Check sheet for the modelled part. Datum: model origin and axes. Units: mm. A direction names the side the tool comes from. Give positions to 0.01 mm unless a question says otherwise; leave off trailing zeros. Order: outer loops, then holes, each group sorted by start corner. A loop starts at its lowest first (then second) coordinate and runs counter-clockwise, first axis right, second up.
Item 1: Sectioned sample at B-B on y = 45.5. Record the boundary of the cut face in (x, z).
Item 2: Access from +Z, -Z, +X, -X, +Y, -Y to the whole of each face (thin tool, end or side, straight path). Record for faces 1 (the flat face through (-117, 30, 88)), 2 (the flat face through (-110, 2, 59)), 3 (the flat face through (107, 70, -92)), 4 (the flat face through (-107, 70, 92)).
Item 3: Sectioned sample at C-C on x = -12.5. Record the boundary of the cut face in (y, z), and give its area (3 significant figures).
Item 4: Sectioned sample at D-D on z = -6. Record the boundary of the cut face in (x, y).
Item 5: Gauge pin test, flat ends, axial feed: P1, Ø10, axis at x = -89.5, z = -13.5, coming from the +Y side; P2, Ø3, axis at x = 94, z = -15, coming from the -Y side. Record the tip position at first contact, or that the pin passes through.
Item 6: Material ranges on line 1 along X through (y, z) = (3.4, 87.5); line 2 along X through (y, z) = (2, 87); line 3 along Y through (x, z) = (98, 87.5), recorded low to high.
Item 7: Sectioned sample at A-A on z = 61.5. Record the boundary of the cut face in (x, y), and give its area (3 significant figures).
Item 8: Release check for a two-part mould opening along X. For faces 5 (the flat face through (125, 76, 0)), 6 (the flat face through (107, 71, 92)), 7 (the flat face through (115, 0, -73)) record: released by +X, released by -X, zero draft, split by the parting line, or undercut.
from build123d import *

# Parameters (mm, degrees)
BOSS_EXTRUDE1_DEPTH   = 100
BOSS_EXTRUDE1_2_DEPTH = 100
BOSS_EXTRUDE1_3_DEPTH = 100
BOSS_EXTRUDE1_4_DEPTH = 100
SKETCH3_W             = 190
SKETCH3_H             = 5
BOSS_EXTRUDE3_DEPTH   = 250
SKETCH5_R             = 2.5
BOSS_EXTRUDE6_DEPTH   = 5
BOSS_EXTRUDE7_DEPTH   = 45
CUT_EXTRUDE2_REACH    = 197.096
CUT_EXTRUDE3_REACH    = 215.454
CUT_EXTRUDE4_REACH    = 197.096
CUT_EXTRUDE5_REACH    = 215.454


with BuildPart() as part:
    # Sketch1 → Boss-Extrude1 (new body)
    with BuildSketch(Plane(origin=(0, 0, 0), x_dir=(1, 0, 0), z_dir=(0, 1, 0))):
        Polygon((-125, 95), (-125, 80), (-110, 95), align=None)
    extrude(amount=BOSS_EXTRUDE1_DEPTH)



with BuildPart() as body_2:
    # Sketch1 → Boss-Extrude1 2 (new body)
    with BuildSketch(Plane(origin=(0, 0, 0), x_dir=(1, 0, 0), z_dir=(0, 1, 0))):
        Polygon((125, 95), (110, 95), (125, 80), align=None)
    extrude(amount=BOSS_EXTRUDE1_2_DEPTH)


with BuildPart() as body_3:
    # Sketch1 → Boss-Extrude1 3 (new body)
    with BuildSketch(Plane(origin=(0, 0, 0), x_dir=(1, 0, 0), z_dir=(0, 1, 0))):
        Polygon((125, -95), (125, -80), (110, -95), align=None)
    extrude(amount=BOSS_EXTRUDE1_3_DEPTH)


with BuildPart() as body_4:
    # Sketch1 → Boss-Extrude1 4 (new body)
    with BuildSketch(Plane(origin=(0, 0, 0), x_dir=(1, 0, 0), z_dir=(0, 1, 0))):
        Polygon((-125, -95), (-110, -95), (-125, -80), align=None)
    extrude(amount=BOSS_EXTRUDE1_4_DEPTH)


with BuildPart() as part_1:
    add(part.part)

    add(body_2.part)  # Boss-Extrude3 merges body 2

    add(body_3.part)  # Boss-Extrude3 merges body 3

    add(body_4.part)  # Boss-Extrude3 merges body 4
    # Sketch3 → Boss-Extrude3 (add, through all)
    with BuildSketch(Plane(origin=(125, 0, 0), x_dir=(0, 0, -1), z_dir=(1, 0, 0))):
        with Locations((0, 77.5)):
            Rectangle(SKETCH3_W, SKETCH3_H)
    extrude(amount=-BOSS_EXTRUDE3_DEPTH)

    # Sketch5 → Boss-Extrude6 (add)
    # profile 1 of 4: a face of its own
    with BuildSketch(Plane.XZ):
        Polygon((-110, 80), (-110, 37.5), (-125, 37.5), (-125, 95), (-67.5, 95), (-67.5, 80), align=None)
        with Locations(Location((-75, 87.5, 0), (0, 0, 270))):
            Circle(SKETCH5_R, mode=Mode.SUBTRACT)
    # profile 2 of 4: a face of its own
    with BuildSketch(Plane.XZ):
        Polygon((125, 95), (67.5, 95), (67.5, 80), (110, 80), (110, 37.5), (125, 37.5), align=None)
        with Locations(Location((75, 87.5, 0), (0, 0, 90))):
            Circle(SKETCH5_R, mode=Mode.SUBTRACT)
    # profile 3 of 4: a face of its own
    with BuildSketch(Plane.XZ):
        Polygon((110, -80), (110, -37.5), (125, -37.5), (125, -95), (67.5, -95), (67.5, -80), align=None)
        with Locations(Location((75, -87.5, 0), (0, 0, 270))):
            Circle(SKETCH5_R, mode=Mode.SUBTRACT)
    # profile 4 of 4: a face of its own
    with BuildSketch(Plane.XZ):
        Polygon((-125, -95), (-67.5, -95), (-67.5, -80), (-110, -80), (-110, -37.5), (-125, -37.5), align=None)
        with Locations(Location((-75, -87.5, 0), (0, 0, 90))):
            Circle(SKETCH5_R, mode=Mode.SUBTRACT)
    extrude(amount=-BOSS_EXTRUDE6_DEPTH)

    # Sketch9 → Boss-Extrude7 (add)
    with BuildSketch(Plane(origin=(0, 100, 0), x_dir=(1, 0, 0), z_dir=(0, 1, 0))):
        Polygon((-110, 95), (-125, 80), (-110.857864376, 65.857864376), (-95.857864376, 80.857864376), align=None)
        Polygon((110, 95), (95.857864376, 80.857864376), (110.857864376, 65.857864376), (125, 80), align=None)
        Polygon((110, -95), (125, -80), (110.857864376, -65.857864376), (95.857864376, -80.857864376), align=None)
        Polygon((-110, -95), (-95.857864376, -80.857864376), (-110.857864376, -65.857864376), (-125, -80), align=None)
    extrude(amount=-BOSS_EXTRUDE7_DEPTH)

    # Sketch11 → Cut-Extrude2 (cut, up to next)
    with BuildSketch(Plane(origin=(7.5, 0, -7.5), x_dir=(0.7071067811865489, 0, 0.7071067811865461), z_dir=(-0.7071067811865461, 0, 0.7071067811865489)), mode=Mode.PRIVATE) as cut_extrude2_sk1:
        with BuildLine():
            Line((124.956890143, 80), (124.956890143, 100))
            Line((124.956890143, 100), (144.956890143, 100))
            ThreePointArc((144.956890143, 100), (139.099025767, 85.857864376), (124.956890143, 80))
        make_face()
    cut_extrude2_tool1 = extrude(cut_extrude2_sk1.sketch, amount=-CUT_EXTRUDE2_REACH, mode=Mode.PRIVATE) & part_1.part
    # Sketch11 → Cut-Extrude2 (cut, up to next)
    with BuildSketch(Plane(origin=(7.5, 0, -7.5), x_dir=(0.7071067811865489, 0, 0.7071067811865461), z_dir=(-0.7071067811865461, 0, 0.7071067811865489)), mode=Mode.PRIVATE) as cut_extrude2_sk2:
        with BuildLine():
            Line((124.956890143, 75), (124.956890143, 55))
            Line((124.956890143, 55), (144.956890143, 55))
            ThreePointArc((144.956890143, 55), (139.099025767, 69.142135624), (124.956890143, 75))
        make_face()
    cut_extrude2_tool2 = extrude(cut_extrude2_sk2.sketch, amount=-CUT_EXTRUDE2_REACH, mode=Mode.PRIVATE) & part_1.part
    add(cut_extrude2_tool1.solids().sort_by_distance((101.859973, 91.511736, 86.859973))[0], mode=Mode.SUBTRACT)
    add(cut_extrude2_tool2.solids().sort_by_distance((101.859973, 63.488264, 86.859973))[0], mode=Mode.SUBTRACT)

    # Sketch12 → Cut-Extrude3 (cut, up to next)
    with BuildSketch(Plane(origin=(22.5, 0, 22.5), x_dir=(0.7071067811865471, 0, -0.7071067811865479), z_dir=(0.7071067811865479, 0, 0.7071067811865471)), mode=Mode.PRIVATE) as cut_extrude3_sk1:
        with BuildLine():
            Line((144.956890143, 100), (124.956890143, 100))
            Line((124.956890143, 100), (124.956890143, 80))
            ThreePointArc((124.956890143, 80), (139.099025767, 85.857864376), (144.956890143, 100))
        make_face()
    cut_extrude3_tool1 = extrude(cut_extrude3_sk1.sketch, amount=-CUT_EXTRUDE3_REACH, mode=Mode.PRIVATE) & part_1.part
    # Sketch12 → Cut-Extrude3 (cut, up to next)
    with BuildSketch(Plane(origin=(22.5, 0, 22.5), x_dir=(0.7071067811865471, 0, -0.7071067811865479), z_dir=(0.7071067811865479, 0, 0.7071067811865471)), mode=Mode.PRIVATE) as cut_extrude3_sk2:
        with BuildLine():
            Line((144.956890143, 55), (124.956890143, 55))
            Line((124.956890143, 55), (124.956890143, 75))
            ThreePointArc((124.956890143, 75), (139.099025767, 69.142135624), (144.956890143, 55))
        make_face()
    cut_extrude3_tool2 = extrude(cut_extrude3_sk2.sketch, amount=-CUT_EXTRUDE3_REACH, mode=Mode.PRIVATE) & part_1.part
    add(cut_extrude3_tool1.solids().sort_by_distance((116.859973, 91.511736, -71.859973))[0], mode=Mode.SUBTRACT)
    add(cut_extrude3_tool2.solids().sort_by_distance((116.859973, 63.488264, -71.859973))[0], mode=Mode.SUBTRACT)

    # Sketch13 → Cut-Extrude4 (cut, up to next)
    with BuildSketch(Plane(origin=(-7.5, 0, -7.5), x_dir=(0.7071067811865482, 0, -0.7071067811865468), z_dir=(0.7071067811865468, 0, 0.7071067811865482)), mode=Mode.PRIVATE) as cut_extrude4_sk1:
        with BuildLine():
            Line((-144.956890143, 100), (-124.956890143, 100))
            Line((-124.956890143, 100), (-124.956890143, 80))
            ThreePointArc((-124.956890143, 80), (-139.099025767, 85.857864376), (-144.956890143, 100))
        make_face()
    cut_extrude4_tool1 = extrude(cut_extrude4_sk1.sketch, amount=-CUT_EXTRUDE4_REACH, mode=Mode.PRIVATE) & part_1.part
    # Sketch13 → Cut-Extrude4 (cut, up to next)
    with BuildSketch(Plane(origin=(-7.5, 0, -7.5), x_dir=(0.7071067811865482, 0, -0.7071067811865468), z_dir=(0.7071067811865468, 0, 0.7071067811865482)), mode=Mode.PRIVATE) as cut_extrude4_sk2:
        with BuildLine():
            Line((-124.956890143, 75), (-124.956890143, 55))
            Line((-124.956890143, 55), (-144.956890143, 55))
            ThreePointArc((-144.956890143, 55), (-139.099025767, 69.142135624), (-124.956890143, 75))
        make_face()
    cut_extrude4_tool2 = extrude(cut_extrude4_sk2.sketch, amount=-CUT_EXTRUDE4_REACH, mode=Mode.PRIVATE) & part_1.part
    add(cut_extrude4_tool1.solids().sort_by_distance((-101.859973, 91.511736, 86.859973))[0], mode=Mode.SUBTRACT)
    add(cut_extrude4_tool2.solids().sort_by_distance((-101.859973, 63.488264, 86.859973))[0], mode=Mode.SUBTRACT)

    # Sketch14 → Cut-Extrude5 (cut, up to next)
    with BuildSketch(Plane(origin=(-22.5, 0, 22.5), x_dir=(0.7071067811865471, 0, 0.7071067811865479), z_dir=(-0.7071067811865479, 0, 0.7071067811865471)), mode=Mode.PRIVATE) as cut_extrude5_sk1:
        with BuildLine():
            Line((-144.956890143, 100), (-124.956890143, 100))
            Line((-124.956890143, 100), (-124.956890143, 80))
            ThreePointArc((-124.956890143, 80), (-139.099025767, 85.857864376), (-144.956890143, 100))
        make_face()
    cut_extrude5_tool1 = extrude(cut_extrude5_sk1.sketch, amount=-CUT_EXTRUDE5_REACH, mode=Mode.PRIVATE) & part_1.part
    # Sketch14 → Cut-Extrude5 (cut, up to next)
    with BuildSketch(Plane(origin=(-22.5, 0, 22.5), x_dir=(0.7071067811865471, 0, 0.7071067811865479), z_dir=(-0.7071067811865479, 0, 0.7071067811865471)), mode=Mode.PRIVATE) as cut_extrude5_sk2:
        with BuildLine():
            Line((-144.956890143, 55), (-124.956890143, 55))
            Line((-124.956890143, 55), (-124.956890143, 75))
            ThreePointArc((-124.956890143, 75), (-139.099025767, 69.142135624), (-144.956890143, 55))
        make_face()
    cut_extrude5_tool2 = extrude(cut_extrude5_sk2.sketch, amount=-CUT_EXTRUDE5_REACH, mode=Mode.PRIVATE) & part_1.part
    add(cut_extrude5_tool1.solids().sort_by_distance((-116.859973, 91.511736, -71.859973))[0], mode=Mode.SUBTRACT)
    add(cut_extrude5_tool2.solids().sort_by_distance((-116.859973, 63.488264, -71.859973))[0], mode=Mode.SUBTRACT)


solid = part_1.part
Report:
1. outline: (-125, -95) - (-110, -95) - (-125, -80) - close; (-125, 80) - (-110, 95) - (-125, 95) - close; (110, -95) - (125, -95) - (125, -80) - close; (110, 95) - (125, 80) - (125, 95) - close
2. face 1: none
2. face 2: -Y
2. face 3: -Z
2. face 4: +Z
3. outline: (75, -95) - (80, -95) - (80, 95) - (75, 95) - close
3. area: 950 mm2
4. outline: (-125, 75) - (125, 75) - (125, 80) - (-125, 80) - close
5. P1: stops at y = 80
5. P2: stops at y = 75
6. line 1: x = -125 to -77.5, -72.5 to -67.5, 67.5 to 72.5, 77.5 to 125
6. line 2: x = -125 to -77.45, -72.55 to -67.5, 67.5 to 72.55, 77.45 to 125
6. line 3: y = 0 to 5, 75 to 80
7. outline: (-125, 0) - (-110, 0) - (-110, 5) - (-125, 5) - close; (-125, 75) - (125, 75) - (125, 80) - (-125, 80) - close; (110, 0) - (125, 0) - (125, 5) - (110, 5) - close
7. area: 1,400 mm2
8. face 5: released by +X
8. face 6: undercut
8. face 7: zero draft
